For this review, take the finished solid that the model builds, in its own axes (mm). A direction names the side the tool comes from. Round coordinates to 2 decimals unless told otherwise and drop trailing zeros. Loops run counter-clockwise (first coordinate to the right, second up) from the corner with the lowest first, then second, coordinate; pieces in that order, holes last. Notation, with made-up numbers: (-36.75, 32.5) -> (-32.75, 32.5) arc R32 cw to (-32.75, 65.5) -> close; hole circle Ø5 at (86.25, 80). An arc over 180 degrees is marked (long way). Use one line per item in the form item = value. Start each with the question number.
from build123d import *

# Parameters (mm, degrees)
SKETCH1_W           = 25.4
SKETCH1_H           = 50.8
SKETCH1_W_2         = 19.05
SKETCH1_H_2         = 44.45
BOSS_EXTRUDE1_DEPTH = 254
CUT_EXTRUDE1_DEPTH  = 149.098


with BuildPart() as part:
    # Sketch1 → Boss-Extrude1 (new body)
    with BuildSketch(Plane(origin=(0, 0, 0), x_dir=(0, 0, -1), z_dir=(1, 0, 0))):
        with Locations((12.7, 25.4)):
            Rectangle(SKETCH1_W, SKETCH1_H)
        with Locations((12.7, 25.4)):
            Rectangle(SKETCH1_W_2, SKETCH1_H_2, mode=Mode.SUBTRACT)
    extrude(amount=BOSS_EXTRUDE1_DEPTH)

    # Sketch2 → Cut-Extrude1 (cut)
    with BuildSketch(Plane(origin=(0, 0, -25.4), x_dir=(-1, 0, 0), z_dir=(0, 0, -1))):
        Polygon((-152.4, 23.345366578), (-152.4, 0), (0, 0), (0, 50.8), (-152.4, 50.8), align=None)
    extrude(amount=-CUT_EXTRUDE1_DEPTH, mode=Mode.SUBTRACT)


solid = part.part
Item 1: Take a section at A-A on y = 26. Give the boundary of the cut face in (x, z) (3 decimals), plus the area to 3 significant figures.
Item 2: Take a section at B-B on z = -21. Give the boundary of the cut face in (x, y) (3 decimals), plus the area to 3 significant figures.
Item 3: Machinability: for faces 1 (the flat face through (202, 25, -22.225)), 2 (the flat face through (152.4, 26, -23)), which of the approach directions +Z, -Z, +X, -X, +Y, -Y give a long, thin tool a straight path to every point of the face, cutting with its end or side? Answer none if there is none.
Item 4: Take a section at C-C on x = 222.5. Give the boundary of the cut face in (y, z) (3 decimals).
Item 5: Wall thickness on line 1 (Y direction, x = 157.5, z = -3.25) (3 decimals); line 2 (Z direction, x = 188.5, y = 21) (3 decimals): over which ranges is each line inside the solid? List them lowest first.
Item 6: Draft analysis for pull direction Y (two halves, no side actions). For faces 3 (the flat face through (202, 25, -3.175)), 4 (the flat face through (202, 50.8, -13)), 5 (the flat face through (202, 0, -13)), 6 (the flat face through (254, 24, -2)), state which applies: +Y half, -Y half, draft (parallel to the pull), parting line (faces both ways), or undercut.
Results:
q1.outline = (152.4, -25.4) -> (254, -25.4) -> (254, -22.225) -> (152.4, -22.225) -> close; (152.4, -3.175) -> (254, -3.175) -> (254, 0) -> (152.4, 0) -> close
q1.area = 645 mm2
q2.outline = (152.4, 0) -> (254, 0) -> (254, 3.175) -> (152.4, 3.175) -> close; (152.4, 47.625) -> (254, 47.625) -> (254, 50.8) -> (152.4, 50.8) -> close
q2.area = 645 mm2
q3.face_1 = +X, -X
q3.face_2 = +Z, -Z, -X, +Y, -Y
q4.outline = (0, -25.4) -> (50.8, -25.4) -> (50.8, 0) -> (0, 0) -> close; hole (3.175, -22.225) -> (47.625, -22.225) -> (47.625, -3.175) -> (3.175, -3.175) -> close
q5.line_1 = 0 to 3.175, 47.625 to 50.8
q5.line_2 = -25.4 to -22.225, -3.175 to 0
q6.face_3 = undercut
q6.face_4 = +Y half
q6.face_5 = -Y half
q6.face_6 = draft
